The listing builds one solid part. Answer for the finished solid, in the listing's coordinates (mm). Face numbers are marked on the shaded views. A direction names the side the tool comes from. Give positions to 0.01 mm unless a question says otherwise; leave off trailing zeros. Write each loop counter-clockwise with the first axis right and the second up, starting at its lowest first coordinate (ties: lowest second). Pieces come first, ordered by that corner, then holes.
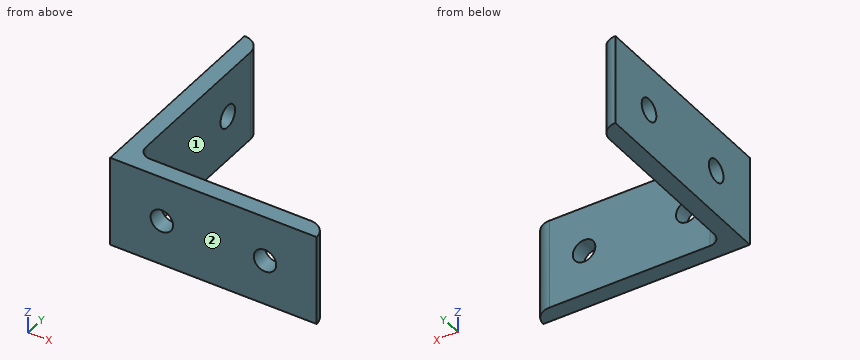
```python
from build123d import *

# Parameters (mm, degrees)
PAD_DEPTH       = 33.33
SKETCH001_R     = 4.15
POCKET_DEPTH    = 76.201
SKETCH002_R     = 4.15
POCKET001_DEPTH = 76.201


with BuildPart() as part:
    # Sketch → Pad (new body)
    with BuildSketch(Plane.XY):
        with BuildLine():
            Line((0, 76.2), (0, 0))
            Line((0, 0), (76.2, 0))
            ThreePointArc((76.2, 0), (74.384062, 4.384062), (70, 6.2))
            Line((10.7, 6.2), (70, 6.2))
            ThreePointArc((6.2, 10.7), (7.518019, 7.518019), (10.7, 6.2))
            Line((6.2, 70), (6.2, 10.7))
            ThreePointArc((6.2, 70), (4.384062, 74.384062), (0, 76.2))
        make_face()
    extrude(amount=PAD_DEPTH)

    # Sketch001 → Pocket (cut, through all)
    with BuildSketch(Plane.XZ):
        with Locations((19.05, 16.665)):
            Circle(SKETCH001_R)
        with Locations((57.15, 16.665)):
            Circle(SKETCH001_R)
    extrude(amount=-POCKET_DEPTH, mode=Mode.SUBTRACT)

    # Sketch002 → Pocket001 (cut, through all)
    with BuildSketch(Plane.YZ):
        with Locations((19.05, 16.665)):
            Circle(SKETCH002_R)
        with Locations((57.15, 16.665)):
            Circle(SKETCH002_R)
    extrude(amount=POCKET001_DEPTH, mode=Mode.SUBTRACT)


solid = part.part
```
Item 1: Each of these flat-tipped pins is pushed along its axis until it touches: P1, Ø10, axis at y = 32.5, z = 24, coming from the +X side; P2, Ø16.5, axis at x = 44.5, z = 19, coming from the +Y side; P3, Ø6.5, axis at x = 19.05, z = 16.665, coming from the -Y side. Where does it stop, or does it pass through?
Conclusion:
P1: stops at x = 6.2
P2: stops at y = 6.2
P3: passes through
Item 2: A cutting plane is placed at C-C, the plane z = 19. Give the vertices of the cut face in (x, y), plus the area to 3 significant figures.
Conclusion:
outline: (0, 0) - (15.62, 0) - (15.62, 6.2) - (10.7, 6.2) arc R4.5 cw to (6.2, 10.7) - (6.2, 15.62) - (0, 15.62) - close; (0, 22.48) - (6.2, 22.48) - (6.2, 53.72) - (0, 53.72) - close; (0, 60.58) - (6.2, 60.58) - (6.2, 70) arc R6.2 ccw to (0, 76.2) - close; (22.48, 0) - (53.72, 0) - (53.72, 6.2) - (22.48, 6.2) - close; (60.58, 0) - (76.2, 0) arc R6.2 ccw to (70, 6.2) - (60.58, 6.2) - close
area: 724 mm2
Item 3: A cutting plane is placed at D-D, the plane z = 3.5. Give the vertices of the cut face in (x, y), plus the area to 3 significant figures.
Conclusion:
outline: (0, 0) - (76.2, 0) arc R6.2 ccw to (70, 6.2) - (10.7, 6.2) arc R4.5 cw to (6.2, 10.7) - (6.2, 70) arc R6.2 ccw to (0, 76.2) - close
area: 894 mm2
Item 4: A cutting plane is placed at A-A, the plane y = 19.05. Give the vertices of the cut face in (x, z) (3 decimals).
Conclusion:
outline: (0, 0) - (6.2, 0) - (6.2, 12.515) - (0, 12.515) - close; (0, 20.815) - (6.2, 20.815) - (6.2, 33.33) - (0, 33.33) - close
Item 5: Which of the six approach directions +Z, -Z, +X, -X, +Y, -Y give full straight-line access (tool end or side, diameter ignored) to the marked faces 1 and 2?
Conclusion:
face 1: +Z, -Z, +X, +Y
face 2: +Z, -Z, +X, -X, -Y
Item 6: Consider probe 1 along Z at (x, y) = (4, 19); probe 2 along Y at (x, z) = (40.5, 10.5). Determine where each line is inside the solid, lowest interval first.
Conclusion:
probe 1: z = 0 to 12.52, 20.81 to 33.33
probe 2: y = 0 to 6.2
